Autodesk Inventor part; units mm, degrees
ref_plane "YZ Plane" through (0, 0, 0) normal (1, 0, 0) x (0, 1, 0)
ref_plane "XZ Plane" through (0, 0, 0) normal (0, 1, 0) x (-1, 0, 0)
ref_plane "XY Plane" through (0, 0, 0) normal (0, 0, 1) x (1, 0, 0)
sketch "Sketch1" plane through (0, 0, 0) normal (0, 0, 1) x (1, 0, 0)
  line L0 (-5, 10) -> (-3.5, 8)
  line L1 (-3.5, 8) -> (-5.5, 8)
  line L2 (5.5, 8) -> (3.5, 8)
  line L3 (3.5, 8) -> (5, 10)
  line L4 (-5.5, 8) -> (-5.5, 6)
  line L5 (5.5, 8) -> (5.5, 6)
  line L6 (-5.5, 6) -> (-2.5, 3)
  line L7 (5.5, 6) -> (2.5, 3)
  line L8 (-2.5, 3) -> (2.5, 3)
  line L9 (-10, 10) -> (-5, 10)
  line L10 (5, 10) -> (10, 10)
  line L11 (3, 2.5) -> (3, -2.5)
  line L12 (3, -2.5) -> (6, -5.5)
  line L13 (6, -5.5) -> (8, -5.5)
  line L14 (8, -5.5) -> (8, -3.5)
  line L15 (8, -3.5) -> (10, -5)
  line L16 (3, 2.5) -> (6, 5.5)
  line L17 (6, 5.5) -> (8, 5.5)
  line L18 (8, 5.5) -> (8, 3.5)
  line L19 (8, 3.5) -> (10, 5)
  line L20 (10, 10) -> (10, 5)
  line L21 (10, -5) -> (10, -10)
  line L22 (-10, 5) -> (-8, 3.5)
  line L23 (-8, 3.5) -> (-8, 5.5)
  line L24 (-8, -5.5) -> (-8, -3.5)
  line L25 (-8, -3.5) -> (-10, -5)
  line L26 (-8, 5.5) -> (-6, 5.5)
  line L27 (-8, -5.5) -> (-6, -5.5)
  line L28 (-6, 5.5) -> (-3, 2.5)
  line L29 (-6, -5.5) -> (-3, -2.5)
  line L30 (-3, 2.5) -> (-3, -2.5)
  line L31 (-10, 10) -> (-10, 5)
  line L32 (-10, -5) -> (-10, -10)
  line L33 (-2.5, -3) -> (2.5, -3)
  line L34 (2.5, -3) -> (5.5, -6)
  line L35 (5.5, -6) -> (5.5, -8)
  line L36 (5.5, -8) -> (3.5, -8)
  line L37 (3.5, -8) -> (5, -10)
  line L38 (-2.5, -3) -> (-5.5, -6)
  line L39 (-5.5, -6) -> (-5.5, -8)
  line L40 (-5.5, -8) -> (-3.5, -8)
  line L41 (-3.5, -8) -> (-5, -10)
  line L42 (-10, -10) -> (-5, -10)
  line L43 (5, -10) -> (10, -10)
  point P0 (0, 0)
  point P1 (0, 0)
  point P2 (0, 0)
  dimension "d0" = 20
  dimension "d1" = 20
  dimension "d3" = 2
  dimension "d4" = 2
  dimension "d6" = 1.5
  dimension "d7" = 2
  dimension "d8" = 2
  dimension "d9" = 3
  dimension "d11" = 3
  dimension "d12" = 3
  dimension "d13" = 5
  dimension "d22" = 5
  dimension "d24" = 3
  dimension "d25" = 3
  dimension "d26" = 2
  dimension "d27" = 5
  dimension "d28" = 2
  dimension "d29" = 2
  dimension "d30" = 1.5
  dimension "d31" = 3
  dimension "d32" = 5
  dimension "d33" = 5
  dimension "d35" = 5
  dimension "d36" = 5
  dimension "d37" = 5
  dimension "d38" = 5
  dimension "d40" = 3
  dimension "d41" = 3
  dimension "d42" = 2
  dimension "d43" = 2
  dimension "d48" = 3
  dimension "d49" = 3
  dimension "d50" = 3
  dimension "d51" = 3
  dimension "d52" = 0.5
  dimension "d53" = 0.5
  dimension "d54" = 0.5
  dimension "d55" = 0.5
  dimension "d56" = 0.5
extrude "Extrusion3" add sketch "Sketch1" along normal blind 100
sketch "Sketch3" plane through (0, 0, 0) normal (0, 0, -1) x (-1, 0, 0)
  circle A0 centre (0, 0) radius 2
  dimension "d59" = 4
extrude "Extrusion4" cut sketch "Sketch3" against normal through all
properties part number "20x20x100 Aluminium VSlot Extrustion"
Can you work these out from the model? Positions are in its coordinate system, mm. A direction names the side the tool comes from. Coordinates: 2 decimals unless noted, no trailing zeros. Order: outer loops, then holes, each group sorted by start corner. A loop starts at its lowest first (then second) coordinate and runs counter-clockwise, first axis right, second up.
1. Thinking about a two-plate mould opening in Y: for faces 1 (the face through (7, 10, 49)), 2 (the face through (5, -8, 49)), 3 (the face through (10, -7, 49)), which applies, +Y half, -Y half, draft (parallel to the pull), parting line (faces both ways), or undercut?
2. If we section it at A-A (y = 0): Please give me the cut outline in (x, z).
3. I'm going to push flat-ended pins straight in: pin 1 (2 mm diameter, centred on y = 2, z = 17, fed in from +X); pin 2 (4 mm diameter, centred on x = -1, z = 35.5, fed in from -Y); pin 3 (1.5 mm diameter, centred on x = 1, z = 46, fed in from +Y). Where does each tip first touch, or does it pass through?
4. I need wall thicknesses on line 1 (Y direction, x = -6.25, z = 55); line 2 (Y direction, x = 0, z = 67.5); line 3 (Y direction, x = -4.25, z = 17). Which ranges of each line are inside material? Lowest first, please.
5. For faces 4 (the face through (-7, 5.5, 49)), 5 (the face through (0, 3, 49)), 6 (the face through (3, 0, 49)), 7 (the face through (0, -3, 49)), which set-ups out of +Z, -Z, +X, -X, +Y, -Y let a thin tool reach every point of the face, with its end or its side?
Entries:
1. face 1: +Y half
1. face 2: undercut
1. face 3: draft
2. outline: (-3, 0) - (-2, 0) - (-2, 100) - (-3, 100) - close; (2, 0) - (3, 0) - (3, 100) - (2, 100) - close
3. pin 1: stops at x = 3.5
3. pin 2: stops at y = -3.5
3. pin 3: stops at y = 3
4. line 1: y = -10 to -5.5, 5.5 to 10
4. line 2: y = -3 to -2, 2 to 3
4. line 3: y = -9 to -8, -4.75 to -3.75, 3.75 to 4.75, 8 to 9
5. face 4: +Z, -Z
5. face 5: +Z, -Z, +Y
5. face 6: +Z, -Z, +X
5. face 7: +Z, -Z, -Y
